Can you work these out from the model? Positions are in its coordinate system, mm. A direction names the side the tool comes from. Round coordinates to 2 decimals unless told otherwise and drop trailing zeros. Loops run counter-clockwise (first coordinate to the right, second up) from the corner with the lowest first, then second, coordinate; pieces in that order, holes last. Notation, with made-up numbers: (76, 80) -> (89, 80) arc R19 cw to (89, 100) -> close; hole circle Ø7 at (-40, -16). An arc over 180 degrees is marked (long way). Write each question's results on one line, items separated by ' | '.
from build123d import *

# Parameters (mm, degrees)
F1_DEPTH     = 17.272
F2_T4_DEPTH  = 145.1755034497
F2_T9_DEPTH  = 145.1755034497
F2_T14_DEPTH = 145.451805042
F2_T19_DEPTH = 145.451805042
F2_T24_DEPTH = 152.4
F2_T29_DEPTH = 152.4
F2_T34_DEPTH = 152.4
F2_T39_DEPTH = 152.4
F2_T45_DEPTH = 152.4
F2_T49_DEPTH = 152.4
F2_T56_DEPTH = 152.4
F2_T60_DEPTH = 152.4


# Not quite as in the source:
# - a fillet or chamfer that OpenCascade refuses, or shapes differently, is made with other operations: its cross-section is extruded or revolved along the edge and cut away or added


with BuildPart() as f1:
    # F0 (on Front) → F1 (new body)
    with BuildSketch(Plane.XZ):
        Polygon((-58.1587258462, 60.3411067049), (-182.2034080142, 87.5792568958), (-182.731828862, 74.8902549096), (-65.2451664209, 51.5867063582), (-65.2451664209, 57.4221499264), (-51.3433068991, 57.4221499264), (-51.3433068991, 51.5329490591), (66.4143771697, 74.8902549096), (65.8859563219, 87.5792568958), align=None)
        Polygon((-65.2451664209, 57.4221499264), (-65.2451664209, 51.5867063582), (-58.1587258462, 50.1811067049), (-51.3433068991, 51.5329490591), (-51.3433068991, 57.4221499264), align=None)
        Polygon((-58.1587258462, 50.1811067049), (-65.2451664209, 51.5867063582), (-65.2451664209, 40.1959307492), (-51.3433068991, 40.1959307492), (-51.3433068991, 51.5329490591), align=None)
    extrude(amount=-F1_DEPTH)

    # F2: fillet of radius 5.08 on 8 edges, made by hand


with BuildPart() as f2_tool2:
    # F2_s3 → F2_t4 (new body)
    with BuildSketch(Plane(origin=(-202.5642945881, 0, 40.1787468945), x_dir=(0, 1, 0), z_dir=(0.9808905749, 0, -0.1945602221))):
        with BuildLine():
            ThreePointArc((12.192, 37.9067999896), (15.7841024484, 39.3946975412), (17.272, 42.9867999896))
            Line((17.272, 42.9867999896), (17.272, 37.9067999896))
            Line((17.272, 37.9067999896), (12.192, 37.9067999896))
        make_face()
    extrude(amount=F2_T4_DEPTH)

    split(bisect_by=Plane.YZ.offset(-65.2451664209), keep=Keep.BOTTOM)


with BuildPart() as f1_1:
    add(f1.part)

    # F2_t1: cut F2_tool2
    add(f2_tool2.part, mode=Mode.SUBTRACT)


with BuildPart() as f2_tool7:
    # F2_s8 → F2_t9 (new body)
    with BuildSketch(Plane(origin=(-202.5642945881, 0, 40.1787468945), x_dir=(0, 1, 0), z_dir=(0.9808905749, 0, -0.1945602221))):
        with BuildLine():
            ThreePointArc((5.08, 37.9067999896), (1.4878975516, 39.3946975412), (0, 42.9867999896))
            Line((0, 42.9867999896), (0, 37.9067999896))
            Line((0, 37.9067999896), (5.08, 37.9067999896))
        make_face()
    extrude(amount=F2_T9_DEPTH)

    split(bisect_by=Plane.YZ.offset(-65.2451664209), keep=Keep.BOTTOM)


with BuildPart() as f1_2:
    add(f1_1.part)

    # F2_t6: cut F2_tool7
    add(f2_tool7.part, mode=Mode.SUBTRACT)


with BuildPart() as f2_tool12:
    # F2_s13 → F2_t14 (new body)
    with BuildSketch(Plane(origin=(-52.0224181794, 0, -10.3186772236), x_dir=(0, 1, 0), z_dir=(0.9808905749, 0, 0.1945602221))):
        with BuildLine():
            ThreePointArc((12.192, 60.5375492231), (15.7841024484, 62.0254467746), (17.272, 65.6175492231))
            Line((17.272, 65.6175492231), (17.272, 60.5375492231))
            Line((17.272, 60.5375492231), (12.192, 60.5375492231))
        make_face()
    extrude(amount=F2_T14_DEPTH)

    split(bisect_by=Plane.YZ.offset(-51.3433068991), keep=Keep.TOP)


with BuildPart() as f1_3:
    add(f1_2.part)

    # F2_t11: cut F2_tool12
    add(f2_tool12.part, mode=Mode.SUBTRACT)


with BuildPart() as f2_tool17:
    # F2_s18 → F2_t19 (new body)
    with BuildSketch(Plane(origin=(-52.0224181794, 0, -10.3186772236), x_dir=(0, 1, 0), z_dir=(0.9808905749, 0, 0.1945602221))):
        with BuildLine():
            ThreePointArc((5.08, 60.5375492231), (1.4878975516, 62.0254467746), (0, 65.6175492231))
            Line((0, 65.6175492231), (0, 60.5375492231))
            Line((0, 60.5375492231), (5.08, 60.5375492231))
        make_face()
    extrude(amount=F2_T19_DEPTH)

    split(bisect_by=Plane.YZ.offset(-51.3433068991), keep=Keep.TOP)


with BuildPart() as f1_4:
    add(f1_3.part)

    # F2_t16: cut F2_tool17
    add(f2_tool17.part, mode=Mode.SUBTRACT)


with BuildPart() as f2_tool22:
    # F2_s23 → F2_t24 (new body)
    with BuildSketch(Plane(origin=(-55.7194406669, 0, 12.2350629379), x_dir=(0, 1, 0), z_dir=(-0.9767297809, 0, 0.2144736236))):
        with BuildLine():
            ThreePointArc((12.192, -46.4634432549), (15.7841024484, -44.9755457034), (17.272, -41.3834432549))
            Line((17.272, -41.3834432549), (17.272, -46.4634432549))
            Line((17.272, -46.4634432549), (12.192, -46.4634432549))
        make_face()
    extrude(amount=F2_T24_DEPTH)

    split(bisect_by=Plane(origin=(-15.3156619604, 0, 69.7487313476), x_dir=(0, 1, 0), z_dir=(-0.2144736236, 0, 0.9767297809)), keep=Keep.TOP)


with BuildPart() as f1_5:
    add(f1_4.part)

    # F2_t21: cut F2_tool22
    add(f2_tool22.part, mode=Mode.SUBTRACT)


with BuildPart() as f2_tool27:
    # F2_s28 → F2_t29 (new body)
    with BuildSketch(Plane(origin=(-55.7194406669, 0, 12.2350629379), x_dir=(0, 1, 0), z_dir=(-0.9767297809, 0, 0.2144736236))):
        with BuildLine():
            ThreePointArc((5.08, -46.4634432549), (1.4878975516, -44.9755457034), (0, -41.3834432549))
            Line((0, -41.3834432549), (0, -46.4634432549))
            Line((0, -46.4634432549), (5.08, -46.4634432549))
        make_face()
    extrude(amount=F2_T29_DEPTH)

    split(bisect_by=Plane(origin=(-15.3156619604, 0, 69.7487313476), x_dir=(0, 1, 0), z_dir=(-0.2144736236, 0, 0.9767297809)), keep=Keep.TOP)


with BuildPart() as f1_6:
    add(f1_5.part)

    # F2_t26: cut F2_tool27
    add(f2_tool27.part, mode=Mode.SUBTRACT)


with BuildPart() as f2_tool32:
    # F2_s33 → F2_t34 (new body)
    with BuildSketch(Plane(origin=(93.6060864991, 0, 20.5543405673), x_dir=(0, 1, 0), z_dir=(-0.9767297809, 0, -0.2144736236))):
        with BuildLine():
            ThreePointArc((5.08, -71.4104686015), (1.4878975516, -69.92257105), (0, -66.3304686015))
            Line((0, -66.3304686015), (0, -71.4104686015))
            Line((0, -71.4104686015), (5.08, -71.4104686015))
        make_face()
    extrude(amount=F2_T34_DEPTH)

    split(bisect_by=Plane(origin=(9.9651830375, 0, 45.382228748), x_dir=(0, 1, 0), z_dir=(0.2144736236, 0, 0.9767297809)), keep=Keep.TOP)


with BuildPart() as f1_7:
    add(f1_6.part)

    # F2_t31: cut F2_tool32
    add(f2_tool32.part, mode=Mode.SUBTRACT)


with BuildPart() as f2_tool37:
    # F2_s38 → F2_t39 (new body)
    with BuildSketch(Plane(origin=(93.6060864991, 0, 20.5543405673), x_dir=(0, 1, 0), z_dir=(-0.9767297809, 0, -0.2144736236))):
        with BuildLine():
            ThreePointArc((12.192, -71.4104686015), (15.7841024484, -69.92257105), (17.272, -66.3304686015))
            Line((17.272, -66.3304686015), (17.272, -71.4104686015))
            Line((17.272, -71.4104686015), (12.192, -71.4104686015))
        make_face()
    extrude(amount=F2_T39_DEPTH)

    split(bisect_by=Plane(origin=(9.9651830375, 0, 45.382228748), x_dir=(0, 1, 0), z_dir=(0.2144736236, 0, 0.9767297809)), keep=Keep.TOP)


with BuildPart() as f1_8:
    add(f1_7.part)

    # F2_t36: cut F2_tool37
    add(f2_tool37.part, mode=Mode.SUBTRACT)


with BuildPart() as f2_tool43:
    # F2_s44 → F2_t45 (new body)
    with BuildSketch(Plane(origin=(93.6060864991, 0, 20.5543405673), x_dir=(0, 1, 0), z_dir=(-0.9767297809, 0, -0.2144736236))):
        with BuildLine():
            ThreePointArc((12.192, -71.4104686015), (15.7841024484, -69.92257105), (17.272, -66.3304686015))
            Line((17.272, -66.3304686015), (17.272, -71.4104686015))
            Line((17.272, -71.4104686015), (12.192, -71.4104686015))
        make_face()
    extrude(amount=F2_T45_DEPTH)

    split(bisect_by=Plane(origin=(9.9651830375, 0, 45.382228748), x_dir=(0, 1, 0), z_dir=(-0.2144736236, 0, -0.9767297809)), keep=Keep.TOP)


with BuildPart() as f2_tool47:
    # F2_s48 → F2_t49 (new body)
    with BuildSketch(Plane(origin=(-55.7194406669, 0, 12.2350629379), x_dir=(0, 1, 0), z_dir=(-0.9767297809, 0, 0.2144736236))):
        with BuildLine():
            ThreePointArc((12.192, -46.4634432549), (15.7841024484, -44.9755457034), (17.272, -41.3834432549))
            Line((17.272, -41.3834432549), (17.272, -46.4634432549))
            Line((17.272, -46.4634432549), (12.192, -46.4634432549))
        make_face()
    extrude(amount=F2_T49_DEPTH)

    split(bisect_by=Plane(origin=(-15.3156619604, 0, 69.7487313476), x_dir=(0, 1, 0), z_dir=(0.2144736236, 0, -0.9767297809)), keep=Keep.TOP)


with BuildPart() as f2_tool43_1:
    add(f2_tool43.part)

    # F2_t51: intersect F2_tool47
    add(f2_tool47.part, mode=Mode.INTERSECT)


with BuildPart() as f1_9:
    add(f1_8.part)

    # F2_t41: cut F2_tool43
    add(f2_tool43_1.part, mode=Mode.SUBTRACT)


with BuildPart() as f2_tool54:
    # F2_s55 → F2_t56 (new body)
    with BuildSketch(Plane(origin=(93.6060864991, 0, 20.5543405673), x_dir=(0, 1, 0), z_dir=(-0.9767297809, 0, -0.2144736236))):
        with BuildLine():
            ThreePointArc((5.08, -71.4104686015), (1.4878975516, -69.92257105), (0, -66.3304686015))
            Line((0, -66.3304686015), (0, -71.4104686015))
            Line((0, -71.4104686015), (5.08, -71.4104686015))
        make_face()
    extrude(amount=F2_T56_DEPTH)

    split(bisect_by=Plane(origin=(9.9651830375, 0, 45.382228748), x_dir=(0, 1, 0), z_dir=(-0.2144736236, 0, -0.9767297809)), keep=Keep.TOP)


with BuildPart() as f2_tool58:
    # F2_s59 → F2_t60 (new body)
    with BuildSketch(Plane(origin=(-55.7194406669, 0, 12.2350629379), x_dir=(0, 1, 0), z_dir=(-0.9767297809, 0, 0.2144736236))):
        with BuildLine():
            ThreePointArc((5.08, -46.4634432549), (1.4878975516, -44.9755457034), (0, -41.3834432549))
            Line((0, -41.3834432549), (0, -46.4634432549))
            Line((0, -46.4634432549), (5.08, -46.4634432549))
        make_face()
    extrude(amount=F2_T60_DEPTH)

    split(bisect_by=Plane(origin=(-15.3156619604, 0, 69.7487313476), x_dir=(0, 1, 0), z_dir=(0.2144736236, 0, -0.9767297809)), keep=Keep.TOP)


with BuildPart() as f2_tool54_1:
    add(f2_tool54.part)

    # F2_t62: intersect F2_tool58
    add(f2_tool58.part, mode=Mode.INTERSECT)


with BuildPart() as f1_10:
    add(f1_9.part)

    # F2_t52: cut F2_tool54
    add(f2_tool54_1.part, mode=Mode.SUBTRACT)


solid = f1_10.part
1. On a 3-axis mill with a long thin cutter (end or side, diameter ignored), from which of +Z, -Z, +X, -X, +Y, -Y can I reach the whole of each face in a straight line? I mean faces 5 (the face through (4.51, 1.53, 72.62)), 6 (the face through (4.73, 8.59, 74.15)), 7 (the face through (-124.92, 1.53, 64.9)). Say none if no direction works.
Final values:
face 5: +Z, -Y | face 6: +Z, +Y, -Y | face 7: -Z, -X, -Y
2. Will these pins go through, and if not, where does the flat tip stop? pin 1 (6 mm diameter, centred on x = 14.5, y = 9.5, fed in from -Z); pin 2 (4 mm diameter, centred on x = -133, z = 67.5, fed in from +Y); pin 3 (10 mm diameter, centred on x = -50.5, y = 12, fed in from -Z); pin 4 (1 mm diameter, centred on y = 9.5, z = 80.5, fed in from -X).
Final values:
pin 1: z = 64 | pin 2: y = 17.23 | pin 3: z = 40.2 | pin 4: x = -182.52
3. If we section it at A-A (y = 14.5): List the corners of the cut face in (x, z) for me, then the cut area to 3 significant figures.
Final values:
outline: (-182.71, 75.45) -> (-65.25, 52.15) -> (-65.25, 40.2) -> (-51.34, 40.2) -> (-51.34, 52.1) -> (66.39, 75.45) -> (65.91, 87.02) -> (-58.16, 59.77) -> (-182.23, 87.02) -> close | area: 2,730 mm2
4. Please list where these lines run through material, in increasing order: line 1 (X direction, y = 9, z = 51.5); line 2 (Y direction, x = -11.5, z = 64.5); line 3 (Z direction, x = 44, y = 7.5). Write a range as from..to.
Final values:
line 1: -65.25..-51.34 | line 2: 0..17.27 | line 3: 70.44..82.77
5. We'd pull the mould along X, two halves only. Please class faces 1 (the face through (-65.245, 9, 47)), 2 (the face through (-119.071, 1.528, 72.233)), 3 (the face through (66.154, 8.515, 81.146)), 4 (the face through (-119.31, 8.59, 73.77)): pulls with the +X half, pulls with the -X half, needs draft (parallel to the pull), parting line crosses it, or undercut.
Final values:
face 1: pulls with the -X half | face 2: undercut | face 3: pulls with the +X half | face 4: undercut
